Verification items for this drawing (mm, ordinates from the low corner). A direction names the side the tool comes from. Round coordinates to 2 decimals unless told otherwise and drop trailing zeros. Loops run counter-clockwise (first coordinate to the right, second up) from the corner with the lowest first, then second, coordinate; pieces in that order, holes last. Notation, with made-up numbers: (3, 15) -> (25, 15) arc R18 cw to (25, 44) -> close; hole circle Ø1 at (10, 86). An arc over 180 degrees is marked (long way). One line per item, written item: value. Start each with the question number.
1. Cross-section at D-D on x = 5. Record the cut outline in (y, z).
2. Cross-section at B-B on z = 4.25. Record the cut outline in (x, y).
3. Go/stop test with flat-tipped pins: pin 1 (2 mm diameter, centred on y = 2.5, z = 1.5, fed in from +X); pin 2 (0.5 mm diameter, centred on x = 8.5, y = 11.5, fed in from +Z); pin 3 (4 mm diameter, centred on y = 5, z = 2, fed in from -X); pin 4 (3 mm diameter, centred on x = 5, y = 10.5, fed in from -Z). Record where each tip stops, or that it passes through.
4. Cross-section at A-A on y = 10.5. Record the cut outline in (x, z), then the cut area to 3 significant figures.
5. Material ranges on L1, parallel to X at y = 14.75, z = 6.5; L2, parallel to Y at x = 5.25, z = 9.25; L3, parallel to Z at x = 8.6, y = 13, recorded low to high.
6. Release check for a two-part mould opening along Y. For the marked faces 1, 2 and 3 record: +Y half, -Y half, draft (parallel to the pull), parting line (faces both ways), or undercut.
7. Cross-section at C-C on x = 8.5. Record the cut outline in (y, z), then the cut area to 3 significant figures.
8. Set-up check for the marked faces 4, 5 and 6: record each of +Z, -Z, +X, -X, +Y, -Y from which the full face is reachable in a straight line by a thin tool's end or side.
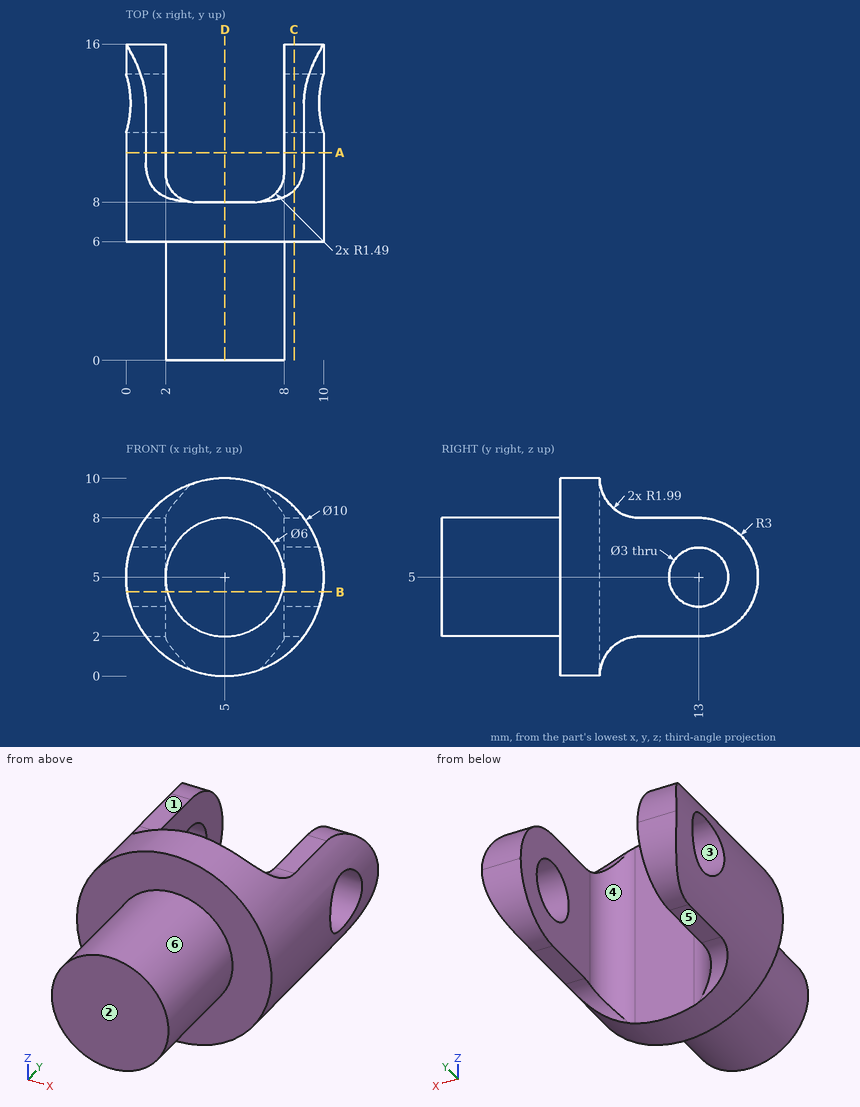
Taken from the geometry:
1. outline: (0, 2) -> (6, 2) -> (6, 0) -> (8, 0) -> (8, 10) -> (6, 10) -> (6, 8) -> (0, 8) -> close
2. outline: (0.06, 6) -> (2.1, 6) -> (2.1, 0) -> (7.9, 0) -> (7.9, 6) -> (9.94, 6) -> (9.94, 11.7) -> (8, 11.7) -> (8, 9.49) arc R1.49 cw to (6.51, 8) -> (3.49, 8) arc R1.49 cw to (2, 9.49) -> (2, 11.7) -> (0.06, 11.7) -> close; (0.06, 14.3) -> (2, 14.3) -> (2, 15.9) -> (0.06, 15.9) -> close; (8, 14.3) -> (9.94, 14.3) -> (9.94, 15.9) -> (8, 15.9) -> close
3. pin 1: stops at x = 6.66
3. pin 2: stops at z = 8
3. pin 3: stops at x = 0.16
3. pin 4: passes through
4. outline: (1, 2) -> (2, 2) -> (2, 8) -> (1, 8) arc R5 ccw to start; (8, 2) -> (9, 2) arc R5 ccw to (9, 8) -> (8, 8) -> close
4. area: 20.2 mm2
5. L1: x = 0.23 to 2, 8 to 9.77
5. L2: y = 6 to 8
5. L3: z = 2 to 3.5, 6.5 to 8
6. face 1: draft
6. face 2: -Y half
6. face 3: undercut
7. outline: (6, 1.43) -> (8.6, 1.43) arc R1.99 cw to (9.99, 2) -> (13, 2) arc R3 ccw to (13, 8) -> (9.99, 8) arc R1.99 cw to (8.6, 8.57) -> (6, 8.57) -> close; hole circle Ø3 at (13, 5)
7. area: 52.5 mm2
8. face 4: +Z, -Z, +Y
8. face 5: -Z, +X, -X, +Y
8. face 6: -Y
